```python
from build123d import *

# Parameters (mm, degrees)
F0_W     = 99.06
F0_H     = 80.01
F0_R     = 35.687
F0_R_2   = 32.639
F1_DEPTH = 4.699
F0_R_3   = 25.527
F2_DEPTH = 4.572


with BuildPart() as f1:
    # F0 (on Top) → F1 (new body)
    with BuildSketch(Plane.XY):
        Rectangle(F0_W, F0_H)
        Circle(F0_R, mode=Mode.SUBTRACT)
        Circle(F0_R)
        Circle(F0_R_2, mode=Mode.SUBTRACT)
    extrude(amount=-F1_DEPTH)

    # F0 (on Top) → F2 (join)
    with BuildSketch(Plane.XY):
        Circle(F0_R)
        Circle(F0_R_2, mode=Mode.SUBTRACT)
        Circle(F0_R_2)
        Circle(F0_R_3, mode=Mode.SUBTRACT)
    extrude(amount=F2_DEPTH)


solid = f1.part
```
Geometry check sheet. Reference: the model listing, model coordinates, mm. A direction names the side the tool comes from. Round coordinates to 2 decimals unless told otherwise and drop trailing zeros. Loops run counter-clockwise (first coordinate to the right, second up) from the corner with the lowest first, then second, coordinate; pieces in that order, holes last. Notation, with made-up numbers: (31, -38.75) -> (50, -38.75) arc R20 ccw to (50, -15.75) -> close; hole circle Ø5 at (52.5, -14.5). An arc over 180 degrees is marked (long way). Use a Markdown table: item, result.
(1) Sectioned sample at C-C (z = -3.5). Enter the section's corners in (x, y) (3 decimals), then the cut area to 3 significant figures.
Calculated:
| item | result |
|---|---|
| outline | (-49.53, -40.005) -> (49.53, -40.005) -> (49.53, 40.005) -> (-49.53, 40.005) -> close; hole circle Ø65.278 at (0, 0) |
| area | 4,580 mm² |
(2) Set-up check for faces 1 (the flat face through (49.53, -1, -2)), 2 (the cylindrical face through (19.19, 30.09, 2.25)), 3 (the flat face through (-19.5, -16.8, 0)): record each of +Z, -Z, +X, -X, +Y, -Y from which the full face is reachable in a straight line by a thin tool's end or side.
Calculated:
| item | result |
|---|---|
| face 1 | +Z, -Z, +X, +Y, -Y |
| face 2 | +Z |
| face 3 | -Z |
(3) Sectioned sample at B-B (x = 0). Enter the section's corners in (y, z) (3 decimals), then the cut area to 3 significant figures.
Calculated:
| item | result |
|---|---|
| outline | (-40.005, -4.699) -> (-32.639, -4.699) -> (-32.639, 0) -> (-25.527, 0) -> (-25.527, 4.572) -> (-35.687, 4.572) -> (-35.687, 0) -> (-40.005, 0) -> close; (25.527, 0) -> (32.639, 0) -> (32.639, -4.699) -> (40.005, -4.699) -> (40.005, 0) -> (35.687, 0) -> (35.687, 4.572) -> (25.527, 4.572) -> close |
| area | 162 mm² |
(4) Go/stop test with a flat-tipped pin: P1, Ø5, axis at x = 20.5, y = -3, coming from the -Z side. Record where the tip stops, or that it passes through.
Calculated:
| item | result |
|---|---|
| P1 | through |
(5) Sectioned sample at D-D (x = 37.5). Enter the section's corners in (y, z) (3 decimals), then the cut area to 3 significant figures.
Calculated:
| item | result |
|---|---|
| outline | (-40.005, -4.699) -> (40.005, -4.699) -> (40.005, 0) -> (-40.005, 0) -> close |
| area | 376 mm² |
(6) Mould release check, pull along X, two halves, no side actions. Record for faces 4 (the cylindrical face through (24.348, 7.668, 2.254)), 5 (the flat face through (-1, 36, 0)), 6 (the flat face through (-49.53, -1, -2)): released by +X, released by -X, zero draft, split by the parting line, or undercut.
Calculated:
| item | result |
|---|---|
| face 4 | undercut |
| face 5 | zero draft |
| face 6 | released by -X |
(7) Sectioned sample at A-A (y = 0). Enter the section's corners in (x, z), then the cut area to 3 significant figures.
Calculated:
| item | result |
|---|---|
| outline | (-49.53, -4.7) -> (-32.64, -4.7) -> (-32.64, 0) -> (-25.53, 0) -> (-25.53, 4.57) -> (-35.69, 4.57) -> (-35.69, 0) -> (-49.53, 0) -> close; (25.53, 0) -> (32.64, 0) -> (32.64, -4.7) -> (49.53, -4.7) -> (49.53, 0) -> (35.69, 0) -> (35.69, 4.57) -> (25.53, 4.57) -> close |
| area | 252 mm² |
(8) Scan lines: probe 1 along X at (y, z) = (-0.5, -3.5); probe 2 along Y at (x, z) = (0.5, 2); probe 3 along Y at (x, z) = (0, -2.3) (3 decimals). Record each from-to range of solid material in increasing order.
Calculated:
| item | result |
|---|---|
| probe 1 | -49.53 to -32.64, 32.64 to 49.53 |
| probe 2 | -35.68 to -25.52, 25.52 to 35.68 |
| probe 3 | -40.005 to -32.639, 32.639 to 40.005 |
